Build history of the part. All positions in model axes, mm. Face numbers are marked on the shaded views. Round coordinates to 2 decimals unless told otherwise and drop trailing zeros. Loops run counter-clockwise (first coordinate to the right, second up) from the corner with the lowest first, then second, coordinate; pieces in that order, holes last. Notation, with made-up numbers: (3, -31) - (45, -31) arc R31 cw to (45, 7) - close; hole circle Ø10 at (44, 52.5). An arc over 180 degrees is marked (long way). One line per question, with ' | ' between items. Start each with the question number.
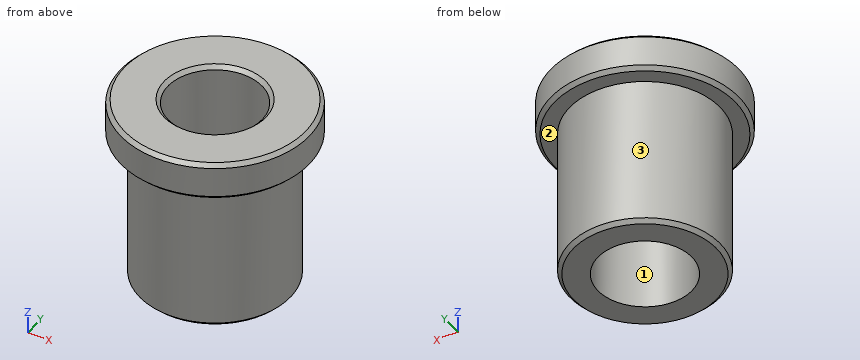
from build123d import *

# Parameters (mm, degrees)
F2_SIZE = 0.2
F3_SIZE = 0.2


with BuildPart() as f1:
    # F0 (on Front) → F1 (revolve)
    with BuildSketch(Plane.XZ):
        Polygon((0, 0), (0, 10), (-2.5, 10), (-2.5, 8), (-1.5, 8), (-1.5, 0), align=None)
    revolve(axis=Axis((2.5, 0, 4.0499057987), (0, 0, -1)))

    # F2
    f2_edges = [f1.edges().sort_by_distance(p)[0] for p in [
        (5, 0, 10),
        (7.5, 0, 10),
    ]]
    chamfer(f2_edges, length=F2_SIZE)

    # F3
    f3_edges = [f1.edges().sort_by_distance(p)[0] for p in [
        (7.5, 0, 8),
        (6.5, 0, 0),
    ]]
    chamfer(f3_edges, length=F3_SIZE)


solid = f1.part
1) Saw through at C-C on z = 6.5. Write the cut outline in (x, y).
2) Two-plate mould, pull along Y, no slides. Class the marked faces 1, 2 and 3: +Y half, -Y half, draft (parallel to the pull), parting line (faces both ways), or undercut.
3) Saw through at A-A on x = 2.5. Write the cut outline in (y, z).
4) Drop flat-ended pins along their axis: pin 1 (3 mm diameter, centred on y = -2.5, z = 3.5, fed in from +X); pin 2 (6 mm diameter, centred on y = -4, z = 8.5, fed in from -X); pin 3 (3 mm diameter, centred on x = -0.5, z = 7, fed in from +Y). Give the stop position or say it passes through.
5) Saw through at B-B on y = 0. Write the cut outline in (x, z).
6) Wall check: line 1 (Y direction, x = 2.5, z = 6.5); line 2 (X direction, y = 0.5, z = 1.25); line 3 (Y direction, x = 3.25, z = 4). Give the ranges that are in metal, low to high. Write a range as [from, to].
Answer key:
1) outline: circle Ø8 at (2.5, 0); hole circle Ø5 at (2.5, 0)
2) face 1: undercut | face 2: draft | face 3: parting line
3) outline: (-5, 8.2) - (-4.8, 8) - (-4, 8) - (-4, 0.2) - (-3.8, 0) - (-2.5, 0) - (-2.5, 9.8) - (-2.7, 10) - (-4.8, 10) - (-5, 9.8) - close; (2.5, 0) - (3.8, 0) - (4, 0.2) - (4, 8) - (4.8, 8) - (5, 8.2) - (5, 9.8) - (4.8, 10) - (2.7, 10) - (2.5, 9.8) - close
4) pin 1: x = 6.37 | pin 2: x = -2.4 | pin 3: y = 4.54
5) outline: (-2.5, 8.2) - (-2.3, 8) - (-1.5, 8) - (-1.5, 0.2) - (-1.3, 0) - (0, 0) - (0, 9.8) - (-0.2, 10) - (-2.3, 10) - (-2.5, 9.8) - close; (5, 0) - (6.3, 0) - (6.5, 0.2) - (6.5, 8) - (7.3, 8) - (7.5, 8.2) - (7.5, 9.8) - (7.3, 10) - (5.2, 10) - (5, 9.8) - close
6) line 1: [-4, -2.5], [2.5, 4] | line 2: [-1.47, 0.05], [4.95, 6.47] | line 3: [-3.93, -2.38], [2.38, 3.93]
